from build123d import *

# Parameters (mm, degrees)
PAD001_DEPTH    = 4
PAD_DEPTH       = 12
POCKET_DEPTH    = 5
PAD002_DEPTH    = 10
POCKET001_DEPTH = 5


with BuildPart() as part:
    # Sketch → Pad001 (new body)
    with BuildSketch(Plane.XY):
        Polygon((19.1896980533, 33.2375320102), (63.1687295291, 55.0322820836), (61.9231008029, 51.9596510451), (20.4096030829, 31.3867489797), (16.9769204172, 33.3686092408), (14.0922142472, 78.735746785), (16.1054778399, 81.7423829), align=None)
    extrude(amount=PAD001_DEPTH)

    # Sketch001 → Pad (join)
    with BuildSketch(Plane.XY):
        Polygon((19.1896980533, 33.2375320102), (60.9462208875, 53.930870371), (61.9231008029, 51.9596510451), (20.1665779687, 31.2663126843), align=None)
    extrude(amount=PAD_DEPTH)

    # Sketch003 (on Face10 of Pad) → Pocket (cut)
    with BuildSketch(Plane(origin=(-9.4403000379, 19.049323856, 0), x_dir=(-0.8960087845, -0.4440363252, 0), z_dir=(-0.4440363252, 0.8960087845, 0))):
        Polygon((-78.5556147914, 12), (-31.9528096, 4), (-31.9528096, 12), align=None)
    extrude(amount=-POCKET_DEPTH, mode=Mode.SUBTRACT)

    # Sketch004 → Pad002 (join)
    with BuildSketch(Plane.XY):
        Polygon((16.2877802175, 78.8753536248), (19.1896980533, 33.2375320102), (16.9941320829, 33.0979251705), (14.0922142472, 78.735746785), align=None)
    extrude(amount=PAD002_DEPTH)

    # Sketch005 (on Face2 of Pad002) → Pocket001 (cut)
    with BuildSketch(Plane(origin=(19.0217824328, 1.209515436, 0), x_dir=(0.0634576544, -0.997984532, 0), z_dir=(-0.997984532, -0.0634576544, 0))):
        Polygon((-31.9528096, 10), (-31.9528096, 8), (-77.6827985443, 10), align=None)
    extrude(amount=-POCKET001_DEPTH, mode=Mode.SUBTRACT)


solid = part.part
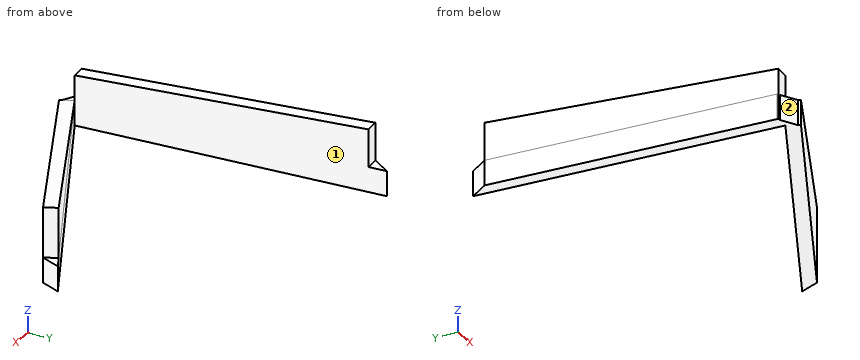
Verification items for the finished model (mm, model axes). Face numbers are marked on the shaded views. Coordinates: 2 decimals unless noted, no trailing zeros. Order: outer loops, then holes, each group sorted by start corner. A loop starts at its lowest first (then second) coordinate and runs counter-clockwise, first axis right, second up. Notation, with made-up numbers: M 36.5,69.25 L 90.5,69.25 A24 ccw 90.5,81.25 Z; hole C 24,10 d4. An arc over 180 degrees is marked long. Return JSON: item names as keys, results as strings.
1) Cross-section at D-D, the plane y = 38. Record the boundary of the cut face in (x, z), and give its area (3 significant figures).
Answer list:
{"outline": "M 16.68,0 L 18.89,0 L 18.89,8.21 L 16.68,8.21 Z; M 28.8,0 L 33.75,0 L 33.75,6.6 L 28.8,5.84 Z", "area": "48.9 mm2"}
2) Gauge pin test, flat ends, axial feed: pin 1 (2 mm diameter, centred on x = 20.5, y = 43, fed in from -Z); pin 2 (6 mm diameter, centred on y = 58, z = 3.5, fed in from -X); pin 3 (0.8 mm diameter, centred on x = 19, y = 32, fed in from +Z); pin 4 (5 mm diameter, centred on y = 64.5, z = 2.5, fed in from -X). Record the tip position at first contact, or that the pin passes through.
Answer list:
{"pin 1": "through", "pin 2": "x = 15.22", "pin 3": "z = 4", "pin 4": "x = 14.84"}
3) Cross-section at A-A, the plane y = 45. Record the boundary of the cut face in (x, z), and give its area (3 significant figures).
Answer list:
{"outline": "M 16.24,0 L 18.44,0 L 18.44,8.52 L 16.24,8.52 Z; M 42.92,0 L 47.88,0 L 47.88,9.31 L 42.92,8.55 Z", "area": "63.0 mm2"}
4) Thickness scan on L1, parallel to X at y = 37, z = 3.5; L2, parallel to X at y = 49, z = 7; L3, parallel to Y at x = 25, z = 3.75. Record the ranges inside material, lowest first. Write a range as [from, to].
Answer list:
{"L1": "[16.75, 18.95], [26.78, 31.74]", "L2": "[15.98, 18.19], [51, 55.95]", "L3": "[33.66, 36.12]"}
5) Cross-section at B-B, the plane z = 5.75. Record the boundary of the cut face in (x, y), and give its area (3 significant figures).
Answer list:
{"outline": "M 14.09,78.74 L 16.99,33.1 L 19.19,33.24 L 16.29,78.88 Z; M 28.32,37.76 L 29.3,35.79 L 61.92,51.96 L 60.95,53.93 Z", "area": "181 mm2"}
6) Release check for a two-part mould opening along X. For the marked faces 1 and 2 record: +X half, -X half, draft (parallel to the pull), parting line (faces both ways), or undercut.
Answer list:
{"face 1": "undercut", "face 2": "-X half"}
7) Cross-section at C-C, the plane z = 1.25. Record the boundary of the cut face in (x, y).
Answer list:
{"outline": "M 14.09,78.74 L 16.99,33.1 L 17.4,33.12 L 19.99,31.63 L 20.17,31.27 L 61.92,51.96 L 63.17,55.03 L 19.19,33.24 L 16.11,81.74 Z"}
